```python
from build123d import *

# Parameters (mm, degrees)
BOSS_EXTRUDE1_DEPTH              = 12.7
CUT_EXTRUDE1_DEPTH               = 13.7
HOLE1_D                          = 30
HOLE1_DEPTH                      = 12.7
HOLE2_D                          = 47
HOLE2_DEPTH                      = 12.7
F_39_0_0995_DIAMETER_HOLE1_D     = 2.5273
F_39_0_0995_DIAMETER_HOLE1_DEPTH = 12.7
F_4_CLEARANCE_HOLE1_D            = 3.3
F_4_CLEARANCE_HOLE1_DEPTH        = 12.7
F_2_CLEARANCE_HOLE1_D            = 2.499999999
F_2_CLEARANCE_HOLE1_DEPTH        = 12.7
F_4_CLEARANCE_HOLE2_D            = 3.3
F_4_CLEARANCE_HOLE2_DEPTH        = 10


with BuildPart() as part:
    # Sketch1 → Boss-Extrude1 (new body)
    with BuildSketch(Plane.XY.offset(12.7)):
        with BuildLine():
            Line((-30, 305), (-30, 23.323807579))
            ThreePointArc((-30, 23.323807579), (0, -38), (30, 23.323807579))
            Line((30, 23.323807579), (30, 305))
            ThreePointArc((30, 305), (0, 335), (-30, 305))
        make_face()
    extrude(amount=-BOSS_EXTRUDE1_DEPTH)

    # Sketch2 → Cut-Extrude1 (cut, through all)
    with BuildSketch(Plane(origin=(0, 0, 0), x_dir=(-1, 0, 0), z_dir=(0, 0, -1))):
        with BuildLine():
            Line((18.5, 74.022471071), (18.5, 84.022471071))
            ThreePointArc((18.5, 84.022471071), (0, 102.522471071), (-18.5, 84.022471071))
            Line((-18.5, 84.022471071), (-18.5, 74.022471071))
            ThreePointArc((-18.5, 74.022471071), (0, 55.522471071), (18.5, 74.022471071))
        make_face()
    extrude(amount=-CUT_EXTRUDE1_DEPTH, mode=Mode.SUBTRACT)

    # Hole1
    with Locations(Plane.XY.offset(12.7)):
        with Locations((0, 0)):
            Hole(HOLE1_D / 2, depth=HOLE1_DEPTH)

    # Hole2
    with Locations(Plane.XY.offset(12.7)):
        with Locations((0, 305)):
            Hole(HOLE2_D / 2, depth=HOLE2_DEPTH)

    # #39 (0.0995) Diameter Hole1
    with Locations(Plane.XY.offset(12.7)):
        with Locations((-26.75, 74.022471071), (-26.75, 129.511235535), (-26.75, 186.111235535), (-26.750000001, 192.911235535), (-26.750000001, 249.511235535), (-26.750000001, 305), (-3.300000001, 331.545668196), (3.299999999, 331.545668196), (26.749999999, 305), (26.749999999, 249.511235535), (26.749999999, 192.911235535), (26.75, 186.111235535), (26.75, 129.511235535), (26.75, 74.022471071), (3.4, 47.489425637), (-3.3, 47.476802874), (-23.166179551, 318.375), (-23.166179551, 291.625), (0, 278.25), (23.166179551, 291.625), (23.166179551, 318.375), (0, 331.75)):
            Hole(F_39_0_0995_DIAMETER_HOLE1_D / 2, depth=F_39_0_0995_DIAMETER_HOLE1_DEPTH)

    # #4 Clearance Hole1
    with Locations(Plane(origin=(0, 0, 0), x_dir=(-1, 0, 0), z_dir=(0, 0, -1))):
        with Locations((-25.5016, 66.772471071), (-25.5016, 91.272471071), (14.424978336, 14.424978336), (20.4, 0), (14.424978336, -14.424978336), (0, -20.4), (-14.424978336, -14.424978336), (-20.4, 0), (-14.424978336, 14.424978336), (0, 20.4), (25.5016, 66.772471071), (25.5016, 91.272471071)):
            Hole(F_4_CLEARANCE_HOLE1_D / 2, depth=F_4_CLEARANCE_HOLE1_DEPTH)

    # #2 Clearance Hole1
    with Locations(Plane(origin=(0, 0, 0), x_dir=(-1, 0, 0), z_dir=(0, 0, -1))):
        with Locations((-1.619921459, 231.265288591), (-21.578861519, 245.43367635)):
            Hole(F_2_CLEARANCE_HOLE1_D / 2, depth=F_2_CLEARANCE_HOLE1_DEPTH)

    # #4 Clearance Hole2
    with Locations(Plane(origin=(30, 0, 0), x_dir=(0, 0, -1), z_dir=(1, 0, 0))):
        with Locations((-6.35, 285.723807579), (-6.35, 133.323807579)):
            Hole(F_4_CLEARANCE_HOLE2_D / 2, depth=F_4_CLEARANCE_HOLE2_DEPTH)


solid = part.part
```
Can you work these out from the model? Positions are in its coordinate system, mm. A direction names the side the tool comes from. Coordinates: 2 decimals unless noted, no trailing zeros. Loops run counter-clockwise (first coordinate to the right, second up) from the corner with the lowest first, then second, coordinate; pieces in that order, holes last.
Item 1: Which directions (+Z, -Z, +X, -X, +Y, -Y) give clear straight access to the entire face, cutting with the end or side of a thin tool? Please do faces 4 (the face through (30, 162, 6)), 5 (the face through (-30, 166, 6)), 6 (the face through (0.407, 55.527, 6.261)).
Answers below:
face 4: +Z, -Z, +X, +Y
face 5: +Z, -Z, -X, +Y
face 6: +Z, -Z
Item 2: If we mould it in two halves opening along Y, with no side actions, what happens to faces 1 (the face through (18.5, 79, 6)), 2 (the face through (-1.19, -37.98, 6.44)), 3 (the face through (-1, 151, 12.7))? For each: released by +Y, released by -Y, zero draft, split by the parting line, or undercut.
Answers below:
face 1: undercut
face 2: split by the parting line
face 3: zero draft
Item 3: Suppose I cut it at D-D (x = 33.5). Please give me the cut outline in (y, z).
Answers below:
outline: (-17.94, 0) - (17.94, 0) - (17.94, 12.7) - (-17.94, 12.7) - close
Item 4: I'm going to push flat-ended pins straight in: pin 1 (5 mm diameter, centred on y = 257, z = 5.5, fed in from +X); pin 2 (2 mm diameter, centred on x = -16, z = 7, fed in from -Y); pin 3 (2 mm diameter, centred on x = -13, z = 8, fed in from +Y). Where does each tip first touch, or does it pass through?
Answers below:
pin 1: stops at x = 30
pin 2: stops at y = -34.91
pin 3: stops at y = 332.5
Item 5: Please list where these lines run through material, in increasing order: L1, parallel to Y at x = 13, z = 6.25; L2, parallel to Y at x = -10, z = 10; L3, parallel to X at y = 66.5, z = 11.5.
Answers below:
L1: y = -35.71 to -15.26, -13.59 to -7.48, 7.48 to 13.59, 15.26 to 60.86, 97.18 to 285.42, 324.58 to 332.04
L2: y = -36.66 to -11.18, 11.18 to 58.46, 99.59 to 283.73, 326.27 to 333.28
L3: x = -30 to -27.13, -23.87 to -16.9, 16.9 to 23.87, 27.13 to 30
Item 6: Suppose I cut it at B-B (y = 98). Please give me the cut outline in (x, z).
Answers below:
outline: (-30, 0) - (-12.12, 0) - (-12.12, 12.7) - (-30, 12.7) - close; (12.12, 0) - (30, 0) - (30, 12.7) - (12.12, 12.7) - close
Item 7: Suppose I cut it at C-C (y = 268.5). Please give me the cut outline in (x, z).
Answers below:
outline: (-30, 0) - (30, 0) - (30, 12.7) - (-30, 12.7) - close
Item 8: Suppose I cut it at A-A (x = 8). Please give me the cut outline in (y, z).
Answers below:
outline: (-37.15, 0) - (-12.69, 0) - (-12.69, 12.7) - (-37.15, 12.7) - close; (12.69, 0) - (57.34, 0) - (57.34, 12.7) - (12.69, 12.7) - close; (100.7, 0) - (282.9, 0) - (282.9, 12.7) - (100.7, 12.7) - close; (327.1, 0) - (333.91, 0) - (333.91, 12.7) - (327.1, 12.7) - close
